Geometry check sheet. Reference: the model listing, model coordinates, mm. Give positions to 0.01 mm unless a question says otherwise; leave off trailing zeros. Order: outer loops, then holes, each group sorted by start corner. A loop starts at its lowest first (then second) coordinate and runs counter-clockwise, first axis right, second up.
from build123d import *

# Parameters (mm, degrees)
BOSS_EXTRUDE1_DEPTH = 107.95
SKETCH2_R           = 2.38125
CUT_EXTRUDE1_DEPTH  = 109.941524835


with BuildPart() as part:
    # Sketch1 → Boss-Extrude1 (new body)
    with BuildSketch(Plane(origin=(0, 0, 0), x_dir=(0, 0, -1), z_dir=(1, 0, 0))):
        Polygon((6.35, -3.666174209), (6.35, 3.666174209), (0, 7.332348419), (-6.35, 3.666174209), (-6.35, -3.666174209), (0, -7.332348419), align=None)
    extrude(amount=BOSS_EXTRUDE1_DEPTH)

    # Sketch2 → Cut-Extrude1 (cut, through all)
    with BuildSketch(Plane.XY.offset(6.35)):
        with Locations((92.5968176, 0)):
            Circle(SKETCH2_R)
    extrude(amount=-CUT_EXTRUDE1_DEPTH, mode=Mode.SUBTRACT)


solid = part.part
Item 1: Sectioned sample at C-C (z = -2.75). Enter the section's corners in (x, y), and give its area (3 significant figures).
Reported:
outline: (0, -5.74) - (107.95, -5.74) - (107.95, 5.74) - (0, 5.74) - close; hole circle Ø4.76 at (92.6, 0)
area: 1,220 mm2
Item 2: Gauge pin test, flat ends, axial feed: pin 1 (2 mm diameter, centred on x = 66.5, z = 0.5, fed in from +Y); pin 2 (1.5 mm diameter, centred on x = 63, z = -3.5, fed in from -Y); pin 3 (3 mm diameter, centred on x = 91, z = -3, fed in from +Y). Record the tip position at first contact, or that the pin passes through.
Reported:
pin 1: stops at y = 7.33
pin 2: stops at y = -5.74
pin 3: stops at y = 6.47
Item 3: Sectioned sample at A-A (y = 0). Enter the section's corners in (x, z), and give its area (3 significant figures).
Reported:
outline: (0, -6.35) - (90.22, -6.35) - (90.22, 6.35) - (0, 6.35) - close; (94.98, -6.35) - (107.95, -6.35) - (107.95, 6.35) - (94.98, 6.35) - close
area: 1,310 mm2
Item 4: Draft check along Y on faces 1 (the flat face through (53.219, 5.474, -3.219)), 2 (the cylindrical face through (94.8, -0.9, 0.1)), 3 (the flat face through (53.219, -5.474, 3.219)), 4 (the flat face through (53, 0, 6.35)). Enter one of: released by +Y, released by -Y, zero draft, split by the parting line, or undercut.
Reported:
face 1: released by +Y
face 2: undercut
face 3: released by -Y
face 4: zero draft
Item 5: Sectioned sample at B-B (x = 15). Enter the section's corners in (y, z), and give its area (3 significant figures).
Reported:
outline: (-7.33, 0) - (-3.67, -6.35) - (3.67, -6.35) - (7.33, 0) - (3.67, 6.35) - (-3.67, 6.35) - close
area: 140 mm2
Item 6: Scan lines: L1, parallel to X at y = -2, z = 3.5; L2, parallel to X at y = 1.5, z = -4.75; L3, parallel to Y at x = 94.5, z = 1 (3 decimals). Record each from-to range of solid material in increasing order.
Reported:
L1: x = 0 to 91.3, 93.89 to 107.95
L2: x = 0 to 90.75, 94.45 to 107.95
L3: y = -6.755 to -1.431, 1.431 to 6.755
